For this review, take the finished solid that the model builds, in its own axes (mm). A direction names the side the tool comes from. Give positions to 0.01 mm unless a question says otherwise; leave off trailing zeros. Loops run counter-clockwise (first coordinate to the right, second up) from the corner with the lowest first, then second, coordinate; pieces in that order, holes last.
```python
from build123d import *

# Parameters (mm, degrees)
SKETCH1_R                   = 6.1341
BOSS_EXTRUDE1_DEPTH         = 19.05
SKETCH2_R                   = 1.53
CUT_EXTRUDE1_DEPTH          = 20.05
F_1_4_20_TAPPED_HOLE1_D     = 5.1054
F_1_4_20_TAPPED_HOLE1_DEPTH = 9.525
F_1_4_20_TAPPED_HOLE1_TIP   = 1.533816902


with BuildPart() as part:
    # Sketch1 → Boss-Extrude1 (new body)
    with BuildSketch(Plane.XY):
        Circle(SKETCH1_R)
    extrude(amount=BOSS_EXTRUDE1_DEPTH)

    # Sketch2 → Cut-Extrude1 (cut, through all)
    with BuildSketch(Plane.XY.offset(19.05)):
        Circle(SKETCH2_R)
    extrude(amount=-CUT_EXTRUDE1_DEPTH, mode=Mode.SUBTRACT)

    # 1/4-20 Tapped Hole1
    with Locations(Plane(origin=(0, 0, 0), x_dir=(-1, 0, 0), z_dir=(0, 0, -1))):
        with Locations((0, 0)):
            Hole(F_1_4_20_TAPPED_HOLE1_D / 2, depth=F_1_4_20_TAPPED_HOLE1_DEPTH)
            with Locations((0, 0, -(F_1_4_20_TAPPED_HOLE1_DEPTH + F_1_4_20_TAPPED_HOLE1_TIP / 2))):  # 118° drill point
                Cone(0, F_1_4_20_TAPPED_HOLE1_D / 2, F_1_4_20_TAPPED_HOLE1_TIP, mode=Mode.SUBTRACT)


solid = part.part
```
Item 1: Take a section at D-D on x = 3. Give the boundary of the cut face in (y, z), and give its area (3 significant figures).
Answer:
outline: (-5.35, 0) - (5.35, 0) - (5.35, 19.05) - (-5.35, 19.05) - close
area: 204 mm2
Item 2: For L1, parallel to Y at x = 0, z = 15; L2, parallel to Y at x = 0, z = 2.75; L3, parallel to X at y = -0.5, z = 18, list the stretches that pass through material, from the lowest coordinate up.
Answer:
L1: y = -6.13 to -1.53, 1.53 to 6.13
L2: y = -6.13 to -2.55, 2.55 to 6.13
L3: x = -6.11 to -1.45, 1.45 to 6.11
Item 3: The part is to be moulded in two halves that separate along X. For faces 3 (the cylindrical face through (5.85, 1.84, 9.39)), 4 (the flat face through (0, -3, 0)), 5 (the cylindrical face through (-0.3, -1.5, 14.7)), say which applies: released by +X, released by -X, zero draft, split by the parting line, or undercut.
Answer:
face 3: split by the parting line
face 4: zero draft
face 5: undercut
Item 4: Clearance check with flat-ended pins moving along their axes: pin 1 Ø1.5 at (x, z) = (-1.5, 8.5) entering from +Y; pin 2 Ø1.5 at (y, z) = (3, 16) entering from -X; pin 3 Ø5 at (y, z) = (-5, 12) entering from -X; pin 4 Ø2.5 at (x, y) = (0, 0) entering from -Z. State where each tip first meets the part, or that it passes through.
Answer:
pin 1: stops at y = 6.09
pin 2: stops at x = -5.71
pin 3: stops at x = -5.6
pin 4: passes through
Item 5: Tool access review of faces 1 (the cylindrical face through (2.435, 0.767, 4.829)), 2 (the flat face through (1.3, -1.3, 19.05)): name each direction out of +Z, -Z, +X, -X, +Y, -Y from which nothing blocks a thin tool from reaching the whole face with its end or side.
Answer:
face 1: -Z
face 2: +Z, +X, -X, +Y, -Y
Item 6: Take a section at C-C on z = 8.5. Give the boundary of the cut face in (x, y), and give its area (3 significant figures).
Answer:
outline: circle Ø12.27 at (0, 0); hole circle Ø5.11 at (0, 0)
area: 97.7 mm2
